The model under review builds one solid part; all positions refer to its coordinate system, in mm. Face numbers are marked on the shaded views. A direction names the side the tool comes from. Give positions to 0.01 mm unless a question says otherwise; leave off trailing zeros. Write each loop counter-clockwise with the first axis right and the second up, starting at its lowest first coordinate (ties: lowest second). Pieces come first, ordered by that corner, then holes. Notation, with made-up numbers: (-8.5, -35) -> (1.5, -35) arc R23 cw to (1.5, -21) -> close; hole circle Ø5 at (24.5, 59.25). An arc over 180 degrees is marked (long way). Use CSV: the item, a comma, the result in double quotes.
```python
from build123d import *

# Parameters (mm, degrees)
SKETCH1_R         = 1.95
SKETCH1_R_2       = 2.15
MAIN_BODY_DEPTH   = 6.91
SKETCH2_R         = 1
TENDON_HOLE_DEPTH = 7.5


with BuildPart() as part:
    # Sketch1 → main body (new body)
    with BuildSketch(Plane.XY):
        with BuildLine():
            Line((8.468803388, 1), (-8.468803388, 1))
            ThreePointArc((-8.468803388, 1), (-14.194141206, 0), (-8.468803388, -1))
            Line((-8.468803388, -1), (8.468803388, -1))
            ThreePointArc((8.468803388, -1), (14.605858794, 0), (8.468803388, 1))
        make_face()
        with Locations((-11.244141206, 0)):
            Circle(SKETCH1_R, mode=Mode.SUBTRACT)
        with Locations((11.455858794, 0)):
            Circle(SKETCH1_R_2, mode=Mode.SUBTRACT)
    extrude(amount=MAIN_BODY_DEPTH)

    # Sketch2 → tendon hole (cut, symmetric)
    with BuildSketch(Plane(origin=(0, 1, 0), x_dir=(1, 0, 0), z_dir=(0, 1, 0))):
        with Locations((11.537331091, -3.455)):
            Circle(SKETCH2_R)
    extrude(amount=TENDON_HOLE_DEPTH, both=True, mode=Mode.SUBTRACT)


solid = part.part
```
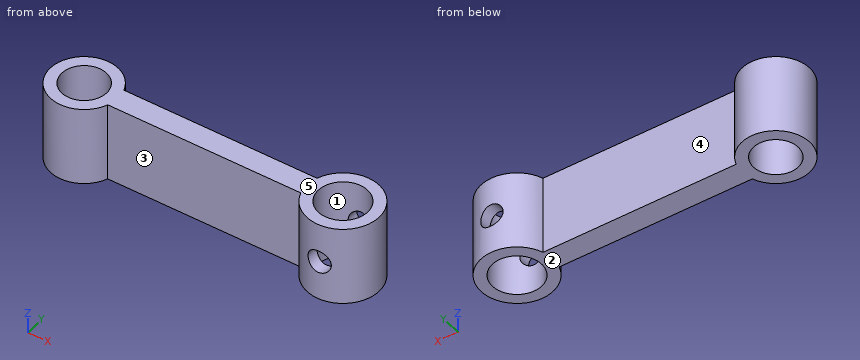
Q1. Machinability: for the marked faces 4 and 5, which of the approach directions +Z, -Z, +X, -X, +Y, -Y give a long, thin tool a straight path to every point of the face, cutting with its end or side? Answer none if there is none.
Derived:
face 4,"+Z, -Z, +Y"
face 5,"+Z, +X, -X, +Y, -Y"
Q2. Consider section B-B (z = 3.75). Write out the cut boundary in (x, y), then the cut area to 3 significant figures.
Derived:
outline,"(-8.47, -1) -> (8.47, -1) arc R3.15 ccw to (10.58, -3.03) -> (10.58, -1.96) arc R2.15 cw to (10.58, 1.96) -> (10.58, 3.03) arc R3.15 ccw to (8.47, 1) -> (-8.47, 1) arc R2.95 ccw (long way) to start; (12.49, -2.97) arc R3.15 ccw to (12.49, 2.97) -> (12.49, 1.88) arc R2.15 cw to (12.49, -1.88) -> close; hole circle Ø3.9 at (-11.24, 0)"
area,"61.6 mm2"
Q3. To check wall thickness, follow probe 1 along X at (y, z) = (0.5, 6); probe 2 along X at (y, z) = (1.75, 5); probe 3 along X at (y, z) = (-2.5, 3.75). State the ranges of each line that lie inside material, in increasing order.
Derived:
probe 1,"x = -14.15 to -13.13, -9.36 to 9.36, 13.55 to 14.57"
probe 2,"x = -13.62 to -12.1, -10.38 to -8.87, 8.84 to 10.21, 12.7 to 14.08"
probe 3,"x = -12.81 to -9.68, 9.54 to 10.58, 12.49 to 13.37"
Q4. The part is to be moulded in two halves that separate along Y. For the marked faces 1, 2 and 3, say which applies: pulls with the +Y half, pulls with the -Y half, needs draft (parallel to the pull), parting line crosses it, or undercut.
Derived:
face 1,"undercut"
face 2,"needs draft"
face 3,"pulls with the -Y half"
Q5. Consider section D-D (z = 1.5). Write out the cut boundary in (x, y), then the cut area to 3 significant figures.
Derived:
outline,"(-8.47, -1) -> (8.47, -1) arc R3.15 ccw (long way) to (8.47, 1) -> (-8.47, 1) arc R2.95 ccw (long way) to start; hole circle Ø3.9 at (-11.24, 0); hole circle Ø4.3 at (11.46, 0)"
area,"65.5 mm2"
Q6. Insertion check: pin 1 (2.5 mm diameter, centred on x = 11.54, z = 3.46, fed in from -Y); pin 2 (1.5 mm diameter, centred on x = -9, z = 5, fed in from -Y); pin 3 (3 mm diameter, centred on y = 2, z = 3, fed in from -X); pin 4 (1 mm diameter, centred on y = -1.5, z = 1, fed in from -X). Each pin has a flat end and moves straight along its axis. Give the tip position at first contact, or say it passes through.
Derived:
pin 1,"stops at y = -3.15"
pin 2,"stops at y = -2.54"
pin 3,"stops at x = -14.15"
pin 4,"stops at x = -14.02"
Q7. Consider section A-A (y = 2.5). Write out the cut boundary in (x, z) (3 decimals), then the cut area to 3 significant figures.
Derived:
outline,"(-12.81, 0) -> (-9.678, 0) -> (-9.678, 6.91) -> (-12.81, 6.91) -> close; (9.539, 0) -> (13.372, 0) -> (13.372, 6.91) -> (9.539, 6.91) -> close; hole circle Ø2 at (11.537, 3.455)"
area,"45.0 mm2"
Q8. Consider section C-C (y = 0). Write out the cut boundary in (x, z), then the cut area to 3 significant figures.
Derived:
outline,"(-14.19, 0) -> (-13.19, 0) -> (-13.19, 6.91) -> (-14.19, 6.91) -> close; (-9.29, 0) -> (9.31, 0) -> (9.31, 6.91) -> (-9.29, 6.91) -> close; (13.61, 0) -> (14.61, 0) -> (14.61, 6.91) -> (13.61, 6.91) -> close"
area,"142 mm2"
